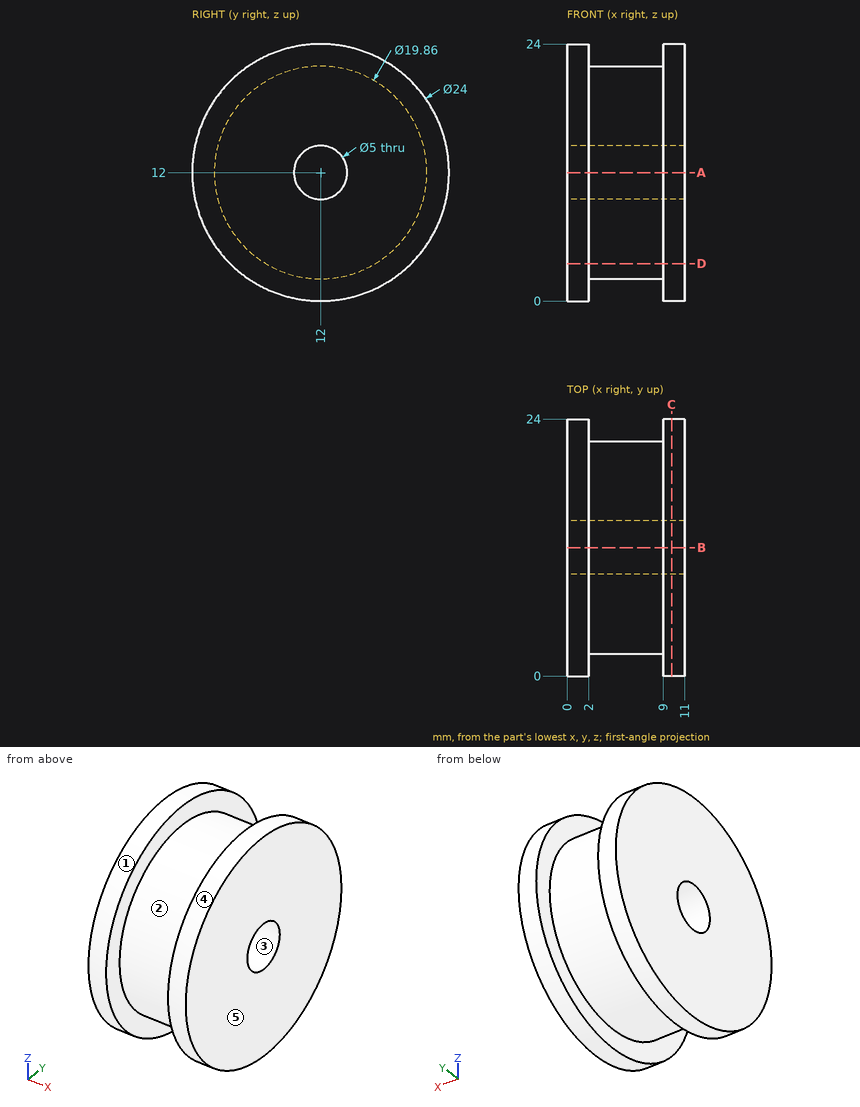
Could you check a few things on this drawing? It's one solid part, dimensions in mm from its lowest x, y, z. A direction names the side the tool comes from. Round coordinates to 2 decimals unless told otherwise and drop trailing zeros. Order: outer loops, then holes, each group sorted by start corner. A loop starts at its lowest first (then second) coordinate and runs counter-clockwise, first axis right, second up. Notation, with made-up numbers: M 15.25,73.5 L 62.25,73.5 A10 cw 62.25,89.5 Z; hole C 65.25,14.25 d3. An arc over 180 degrees is marked long. One line per item, written item: value.
(1) Imagine slicing it at D-D (z = 3.5). Write out the boundary of the cut face in (x, y), and give its area (3 significant figures).
Ans:
outline: M 0,3.53 L 2,3.53 L 2,6.87 L 9,6.87 L 9,3.53 L 11,3.53 L 11,20.47 L 9,20.47 L 9,17.13 L 2,17.13 L 2,20.47 L 0,20.47 Z
area: 140 mm^2
(2) I'm going to push flat-ended pins straight in: P1, Ø3, axis at y = 6.5, z = 3, coming from the -X side; P2, Ø1.5, axis at x = 8, z = 13, coming from the -Y side; P3, Ø6, axis at x = 8, z = 17.5, coming from the -Y side; P4, Ø6, axis at x = 6.5, z = 9, coming from the -Y side. Where does each tip first touch, or does it pass through?
Ans:
P1: stops at x = 0
P2: stops at y = 2.07
P3: stops at y = 0.3
P4: stops at y = 0.08
(3) Imagine slicing it at C-C (x = 9.75). Write out the boundary of the cut face in (y, z), and give its area (3 significant figures).
Ans:
outline: C 12,12 d24; hole C 12,12 d5
area: 433 mm^2
(4) If we mould it in two halves opening along Z, with no side actions, what happens to the marked faces 3, 4 and 5? For each: released by +Z, released by -Z, zero draft, split by the parting line, or undercut.
Ans:
face 3: undercut
face 4: split by the parting line
face 5: zero draft
(5) Imagine slicing it at A-A (z = 12). Write out the boundary of the cut face in (x, y).
Ans:
outline: M 0,0 L 2,0 L 2,2.07 L 9,2.07 L 9,0 L 11,0 L 11,9.5 L 0,9.5 Z; M 0,14.5 L 11,14.5 L 11,24 L 9,24 L 9,21.93 L 2,21.93 L 2,24 L 0,24 Z
(6) I need wall thicknesses on line 1 along Z through (x, y) = (3.5, 12); line 2 along X through (y, z) = (15.5, 22); line 3 along Y through (x, z) = (3.75, 5.5). Which ranges of each line are inside material? Lowest first, please. Write a range as from..to.
Ans:
line 1: z = 2.07..9.5, 14.5..21.93
line 2: x = 0..2, 9..11
line 3: y = 4.49..19.51
(7) Which directions (+Z, -Z, +X, -X, +Y, -Y) give clear straight access to the entire face, cutting with the end or side of a thin tool? Please do the marked faces 1 and 2.
Ans:
face 1: +X, -X
face 2: none
